The model under review builds one solid part; all positions refer to its coordinate system, in mm. Give positions to 0.01 mm unless a question says otherwise; leave off trailing zeros. Order: outer loops, then holes, each group sorted by start corner. A loop starts at its lowest first (then second) coordinate and runs counter-clockwise, first axis right, second up. Notation, with made-up numbers: (53.25, 47.25) -> (57.25, 47.25) arc R11 cw to (57.25, 53.25) -> close; hole circle Ø8 at (25, 6). An arc over 180 degrees is marked (long way). Use one line per item in the form item = value.
```python
from build123d import *

# Parameters (mm, degrees)
MODEL_W             = 26.170325549
MODEL_H             = 4.242293888
MODEL_W_2           = 26.212023883
MODEL_H_2           = 4.119633054
BOSS_EXTRUDE1_DEPTH = 4.5


with BuildPart() as part:
    # Model → Boss-Extrude1 (new body)
    with BuildSketch(Plane.XY):
        with BuildLine():
            Line((1149.554293324, -552.580562917), (1145.054295269, -552.580562917))
            Line((1145.054295269, -552.580562917), (1145.054295269, -527.830661812))
            Line((1145.054295269, -527.830661812), (1166.254405264, -527.830661812))
            add(Edge.make_bspline(
                [(1198.054358589, -527.830661812), (1180.491599149, -527.830661812), (1166.254405264, -527.830661812)],
                knots=[1, 1, 1, 2, 2, 2], degree=2))
            add(Edge.make_bspline(
                [(1229.854311915, -527.830661812), (1215.617118029, -527.830661812), (1198.054358589, -527.830661812)],
                knots=[0, 0, 0, 1, 1, 1], degree=2))
            Line((1229.854311915, -527.830661812), (1251.054386632, -527.830661812))
            Line((1251.054386632, -527.830661812), (1251.054386632, -552.580562917))
            Line((1251.054386632, -552.580562917), (1246.554388577, -552.580562917))
            Line((1246.554388577, -552.580562917), (1246.554388577, -581.830462077))
            Line((1246.554388577, -581.830462077), (1251.054386632, -581.830462077))
            Line((1251.054386632, -581.830462077), (1251.054386632, -602.83072346))
            Line((1251.054386632, -602.83072346), (1246.554388577, -602.83072346))
            Line((1246.554388577, -602.83072346), (1246.554388577, -623.830667344))
            Line((1246.554388577, -623.830667344), (1251.054386632, -623.830667344))
            Line((1251.054386632, -623.830667344), (1251.054386632, -644.83057595))
            Line((1251.054386632, -644.83057595), (1246.554388577, -644.83057595))
            Line((1246.554388577, -644.83057595), (1246.554388577, -665.830519834))
            Line((1246.554388577, -665.830519834), (1251.054386632, -665.830519834))
            Line((1251.054386632, -665.830519834), (1251.054386632, -686.830428439))
            Line((1251.054386632, -686.830428439), (1246.554388577, -686.830428439))
            Line((1246.554388577, -686.830428439), (1246.554388577, -707.830689823))
            Line((1246.554388577, -707.830689823), (1251.054386632, -707.830689823))
            Line((1251.054386632, -707.830689823), (1251.054386632, -729.002718707))
            Line((1251.054386632, -729.002718707), (1246.554388577, -729.002718707))
            Line((1246.554388577, -729.002718707), (1246.554388577, -825.00268896))
            Line((1246.554388577, -825.00268896), (1229.854311915, -825.00268896))
            Line((1229.854311915, -825.00268896), (1229.854311915, -829.502687015))
            Line((1229.854311915, -829.502687015), (1208.654554698, -829.502687015))
            Line((1208.654554698, -829.502687015), (1208.654554698, -825.00268896))
            Line((1208.654554698, -825.00268896), (1199.604287756, -825.00268896))
            Line((1199.604287756, -825.00268896), (1196.504394145, -825.00268896))
            Line((1196.504394145, -825.00268896), (1187.454127203, -825.00268896))
            Line((1187.454127203, -825.00268896), (1187.454127203, -829.502687015))
            Line((1187.454127203, -829.502687015), (1166.254405264, -829.502687015))
            Line((1166.254405264, -829.502687015), (1166.254405264, -825.00268896))
            Line((1166.254405264, -825.00268896), (1149.554293324, -825.00268896))
            Line((1149.554293324, -825.00268896), (1149.554293324, -729.002718707))
            Line((1149.554293324, -729.002718707), (1145.054295269, -729.002718707))
            Line((1145.054295269, -729.002718707), (1145.054295269, -707.911123156))
            Line((1145.054295269, -707.911123156), (1149.554293324, -707.911123156))
            Line((1149.554293324, -707.911123156), (1149.554293324, -686.830428439))
            Line((1149.554293324, -686.830428439), (1145.054295269, -686.830428439))
            Line((1145.054295269, -686.830428439), (1145.054295269, -665.830519834))
            Line((1145.054295269, -665.830519834), (1149.554293324, -665.830519834))
            Line((1149.554293324, -665.830519834), (1149.554293324, -644.83057595))
            Line((1149.554293324, -644.83057595), (1145.054295269, -644.83057595))
            Line((1145.054295269, -644.83057595), (1145.054295269, -623.830667344))
            Line((1145.054295269, -623.830667344), (1149.554293324, -623.830667344))
            Line((1149.554293324, -623.830667344), (1149.554293324, -602.83072346))
            Line((1149.554293324, -602.83072346), (1145.054295269, -602.83072346))
            Line((1145.054295269, -602.83072346), (1145.054295269, -581.830462077))
            Line((1145.054295269, -581.830462077), (1149.554293324, -581.830462077))
            Line((1149.554293324, -581.830462077), (1149.554293324, -552.580562917))
        make_face()
        with Locations((1227.987059138, -738.28775926)):
            Rectangle(MODEL_W, MODEL_H, mode=Mode.SUBTRACT)
        with Locations((1168.453233875, -738.287741621)):
            Rectangle(MODEL_W_2, MODEL_H_2, mode=Mode.SUBTRACT)
        with BuildLine():
            add(Edge.make_bspline(
                [(1183.054388593, -780.523584805), (1183.054388593, -772.239339529), (1189.770254425, -765.523650086), (1198.054358589, -765.523650086), (1206.338427476, -765.523650086), (1213.054293308, -772.239339529), (1213.054293308, -780.523584805)],
                knots=[2, 2, 2, 2, 3, 3, 3, 4, 4, 4, 4], degree=3))
            add(Edge.make_bspline(
                [(1213.054293308, -780.523584805), (1213.054293308, -788.807830081), (1206.338427476, -795.523519523), (1198.054358589, -795.523519523), (1189.770254425, -795.523519523), (1183.054388593, -788.807830081), (1183.054388593, -780.523584805)],
                knots=[0, 0, 0, 0, 1, 1, 1, 2, 2, 2, 2], degree=3))
        make_face(mode=Mode.SUBTRACT)
    extrude(amount=BOSS_EXTRUDE1_DEPTH)


solid = part.part
```
1. Add section B-B on y = -697.5. Give the boundary of the cut face in (x, z).
Values:
outline = (1149.55, 0) -> (1246.55, 0) -> (1246.55, 4.5) -> (1149.55, 4.5) -> close
2. Add section A-A on z = 2.4. Count the separate pieces of the cut face and the enclosed holes in it, then the cut area to 3 significant figures.
Values:
separate_pieces = 1
enclosed_holes = 3
area = 29,100 mm^2
3. For L1, parallel to X at y = -740, z = 3; L2, parallel to Y at x = 1171, z = 2.9; L3, parallel to Y at x = 1234, z = 1.25, list the stretches that pass through material, from the lowest coordinate up.
Values:
L1 = 1149.55 to 1155.35, 1181.56 to 1214.9, 1241.07 to 1246.55
L2 = -829.5 to -740.35, -736.23 to -527.83
L3 = -825 to -740.41, -736.17 to -527.83
4. For pin 1 Ø1.3 at (x, z) = (1148, 3.5) entering from -Y; pin 2 Ø2 at (y, z) = (-562.5, 1.5) entering from -X; pin 3 Ø2 at (y, z) = (-755.5, 1) entering from +X, all flat-tipped, find the tip position at first contact; note any pin that passes through.
Values:
pin_1 = -729
pin_2 = 1149.55
pin_3 = 1246.55
